Design review of the part built by this model. Coordinates are the model's own, in mm. A direction names the side the tool comes from. Coordinates: 2 decimals unless noted, no trailing zeros. Write each loop counter-clockwise with the first axis right and the second up, starting at its lowest first coordinate (ties: lowest second). Pieces come first, ordered by that corner, then holes. Notation, with made-up numbers: (-34.75, 4.5) - (20.25, 4.5) arc R20 cw to (20.25, 24.5) - close; hole circle Ø5 at (-5, 5). An arc over 180 degrees is marked (long way). Use a Markdown table: item, result.
Autodesk Inventor part; units mm, degrees
ref_plane "YZ Plane" through (0, 0, 0) normal (1, 0, 0) x (0, 1, 0)
ref_plane "XZ Plane" through (0, 0, 0) normal (0, 1, 0) x (-1, 0, 0)
ref_plane "XY Plane" through (0, 0, 0) normal (0, 0, 1) x (1, 0, 0)
sketch "Sketch1" plane through (0, 0, 0) normal (0, 0, 1) x (1, 0, 0)
  line L0 (-37.6, -18) -> (37.6, -18)
  line L1 (37.6, -18) -> (37.6, 18)
  line L2 (37.6, 18) -> (-37.6, 18)
  line L3 (-37.6, 18) -> (-37.6, -18)
  line L4 (-37.6, -18) -> (37.6, 18) construction
  line L5 (37.6, -18) -> (-37.6, 18) construction
  line L6 (-15.1, 18) -> (5.2739, 18)
  line L7 (-14.8, -18) -> (-37.6, -18)
  line L8 (-37.6, -18) -> (-37.6, -13)
  line L9 (0, 0) -> (0, -18) construction
  line L10 (14.8, -18) -> (37.6, -18)
  line L11 (37.6, -18) -> (37.6, -13)
  line L12 (-15.1, 18) -> (-37.6, 18)
  line L13 (-37.6, 18) -> (-37.6, 13)
  line L14 (15.1, 18) -> (37.6, 18)
  line L15 (37.6, 18) -> (37.6, 13)
  line L16 (-15, -13) -> (15, -13) construction
  line L17 (15, -13) -> (15, -18)
  line L18 (15, -18) -> (-15, -18)
  line L19 (-15, -18) -> (-15, -13)
  line L20 (-15, -13) -> (15, -18) construction
  line L21 (15, -13) -> (-15, -18) construction
  line L22 (-15, -13) -> (-37.6, -13)
  line L23 (15, -13) -> (37.6, -13)
  line L24 (-37.6, 13) -> (-15.6, 13) construction
  line L25 (-15.6, 13) -> (-15.6, 18)
  line L26 (-15.6, 18) -> (-37.6, 18)
  line L27 (-37.6, 18) -> (-37.6, 13)
  line L28 (-37.6, 13) -> (-15.6, 18) construction
  line L29 (-15.6, 13) -> (-37.6, 18) construction
  line L30 (15.6, 13) -> (37.6, 13) construction
  line L31 (37.6, 13) -> (37.6, 18)
  line L32 (37.6, 18) -> (15.6, 18)
  line L33 (15.6, 18) -> (15.6, 13)
  line L34 (15.6, 13) -> (37.6, 18) construction
  line L35 (37.6, 13) -> (15.6, 18) construction
  line L36 (-15.6, 13) -> (15.6, 13)
  point P0 (0, -15.5)
  point P1 (-37.6, -13)
  point P2 (-15, -18)
  point P3 (-26.6, 15.5)
  point P4 (26.6, 15.5)
  point P5 (15.6, 18)
  dimension "d1" = 36
  dimension "d27" = 5
  dimension "d28" = 30
  dimension "d30" = 5
  dimension "d31" = 5
  dimension "d32" = 22
  dimension "d33" = 22
  dimension "d34" = 53.2
extrude "Extrusion1" add sketch "Sketch1" along normal blind 5 contours L19 L22 L3 L2 L25 L36 L33 L1 L23 L17 L0
equation "\"d31\" = d30"
equation "\"d33\" = d32"
properties part number "lower-back-plate-support"
(1) Machinability: for faces 1 (the flat face through (0, 13, 2)), 2 (the flat face through (26, -13, 2)), 3 (the flat face through (-26, -13, 2)), which of the approach directions +Z, -Z, +X, -X, +Y, -Y give a long, thin tool a straight path to every point of the face, cutting with its end or side? Answer none if there is none.
Determined:
| item | result |
|---|---|
| face 1 | +Z, -Z, +Y |
| face 2 | +Z, -Z, +X, -Y |
| face 3 | +Z, -Z, -X, -Y |
(2) For pin 1 (2.5 mm diameter, centred on x = 21.5, z = 2, fed in from -Y); pin 2 (1 mm diameter, centred on x = -14.5, z = 1, fed in from +Y); pin 3 (1.5 mm diameter, centred on y = -15.5, z = 3, fed in from +X), all flat-tipped, find the tip position at first contact; note any pin that passes through.
Determined:
| item | result |
|---|---|
| pin 1 | y = -13 |
| pin 2 | y = 13 |
| pin 3 | x = 15 |
(3) Take a section at B-B on z = 2.85. Write out the cut boundary in (x, y).
Determined:
| item | result |
|---|---|
| outline | (-37.6, -13) - (-15, -13) - (-15, -18) - (15, -18) - (15, -13) - (37.6, -13) - (37.6, 18) - (15.6, 18) - (15.6, 13) - (-15.6, 13) - (-15.6, 18) - (-37.6, 18) - close |
(4) Take a section at A-A on y = 14. Write out the cut boundary in (x, z), and give its area (3 significant figures).
Determined:
| item | result |
|---|---|
| outline | (-37.6, 0) - (-15.6, 0) - (-15.6, 5) - (-37.6, 5) - close; (15.6, 0) - (37.6, 0) - (37.6, 5) - (15.6, 5) - close |
| area | 220 mm2 |
(5) Draft analysis for pull direction Z (two halves, no side actions). For faces 4 (the flat face through (-1, 0, 5)), 5 (the flat face through (-1, 0, 0)), 6 (the flat face through (15, -15, 2)), state which applies: +Z half, -Z half, draft (parallel to the pull), parting line (faces both ways), or undercut.
Determined:
| item | result |
|---|---|
| face 4 | +Z half |
| face 5 | -Z half |
| face 6 | draft |
(6) For L1, parallel to Y at x = 8, z = 0.8; L2, parallel to Y at x = -18, z = 1.7; L3, parallel to X at y = 15, z = 3.1, list the stretches that pass through material, from the lowest coordinate up. Write a range as from..to.
Determined:
| item | result |
|---|---|
| L1 | -18..13 |
| L2 | -13..18 |
| L3 | -37.6..-15.6, 15.6..37.6 |
(7) Take a section at C-C on x = -26. Write out the cut boundary in (y, z).
Determined:
| item | result |
|---|---|
| outline | (-13, 0) - (18, 0) - (18, 5) - (-13, 5) - close |
(8) Take a section at D-D on y = -15. Write out the cut boundary in (x, z).
Determined:
| item | result |
|---|---|
| outline | (-15, 0) - (15, 0) - (15, 5) - (-15, 5) - close |
